Geometry check sheet. Reference: the model listing, model coordinates, mm. A direction names the side the tool comes from. Give positions to 0.01 mm unless a question says otherwise; leave off trailing zeros. Order: outer loops, then holes, each group sorted by start corner. A loop starts at its lowest first (then second) coordinate and runs counter-clockwise, first axis right, second up.
from build123d import *

# Parameters (mm, degrees)
SKETCH1_R           = 1.55
BOSS_EXTRUDE1_DEPTH = 1.5748
SKETCH2_W           = 12.4
SKETCH2_H           = 28.6
BOSS_EXTRUDE2_DEPTH = 24.9
SKETCH3_W           = 4.75
SKETCH3_H           = 0.5
BOSS_EXTRUDE3_DEPTH = 8.5
SKETCH4_W           = 45
SKETCH4_H           = 57.9
BOSS_EXTRUDE4_DEPTH = 19.1


with BuildPart() as part:
    # Sketch1 → Boss-Extrude1 (new body)
    with BuildSketch(Plane.XY):
        with BuildLine():
            Line((42.354093023, -30.703264053), (42.354093023, -32.943264053))
            Line((42.354093023, -32.943264053), (-42.354093023, -32.943264053))
            Line((-42.354093023, -32.943264053), (-42.354093023, -30.703264053))
            ThreePointArc((-42.354093023, -30.703264053), (-45.283025211, -23.632196241), (-52.354093023, -20.703264053))
            Line((-52.354093023, -20.703264053), (-60.301272865, -20.703264053))
            Line((-60.301272865, -20.703264053), (-60.301272865, 20.296735947))
            Line((-60.301272865, 20.296735947), (-52.354093023, 20.296735947))
            ThreePointArc((-52.354093023, 20.296735947), (-45.283025211, 23.225668135), (-42.354093023, 30.296735947))
            Line((-42.354093023, 30.296735947), (-42.354093023, 32.536735947))
            Line((-42.354093023, 32.536735947), (42.354093023, 32.536735947))
            Line((42.354093023, 32.536735947), (42.354093023, 30.296735947))
            ThreePointArc((42.354093023, 30.296735947), (45.283025211, 23.225668135), (52.354093023, 20.296735947))
            Line((52.354093023, 20.296735947), (54.593335979, 20.296735947))
            Line((54.593335979, 20.296735947), (54.593335979, -20.703264053))
            Line((54.593335979, -20.703264053), (52.354093023, -20.703264053))
            ThreePointArc((52.354093023, -20.703264053), (45.283025211, -23.632196241), (42.354093023, -30.703264053))
        make_face()
        with Locations((49.618335979, -15.728264053)):
            Circle(SKETCH1_R, mode=Mode.SUBTRACT)
        with Locations((49.618335979, 15.321735947)):
            Circle(SKETCH1_R, mode=Mode.SUBTRACT)
    extrude(amount=BOSS_EXTRUDE1_DEPTH)

    # Sketch2 → Boss-Extrude2 (add)
    with BuildSketch(Plane.XY.offset(1.5748)):
        with Locations((-30.457181744, 14.174173465)):
            Rectangle(SKETCH2_W, SKETCH2_H)
        with Locations((-16.057181744, 14.174173465)):
            Rectangle(SKETCH2_W, SKETCH2_H)
    extrude(amount=BOSS_EXTRUDE2_DEPTH)

    # Sketch3 → Boss-Extrude3 (add)
    with BuildSketch(Plane.XY.offset(26.4748)):
        with Locations((-16.064182879, 4.152019918)):
            Rectangle(SKETCH3_W, SKETCH3_H)
        with Locations((-16.064182879, 10.652019918)):
            Rectangle(SKETCH3_W, SKETCH3_H)
        with Locations((-30.792693371, 4.152019918)):
            Rectangle(SKETCH3_W, SKETCH3_H)
        with Locations((-30.792693371, 10.652019918)):
            Rectangle(SKETCH3_W, SKETCH3_H)
    extrude(amount=BOSS_EXTRUDE3_DEPTH)

    # Sketch4 → Boss-Extrude4 (add)
    with BuildSketch(Plane.XY.offset(1.5748)):
        with Locations((15.786645431, 0.061567403)):
            Rectangle(SKETCH4_W, SKETCH4_H)
    extrude(amount=BOSS_EXTRUDE4_DEPTH)


solid = part.part
Item 1: Sectioned sample at C-C (y = -3). Enter the section's corners in (x, z), and give its area (3 significant figures).
Reported:
outline: (-60.3, 0) - (54.59, 0) - (54.59, 1.57) - (38.29, 1.57) - (38.29, 20.67) - (-6.71, 20.67) - (-6.71, 1.57) - (-60.3, 1.57) - close
area: 1,040 mm2
Item 2: Sectioned sample at D-D (x = 30). Enter the section's corners in (y, z), and give its area (3 significant figures).
Reported:
outline: (-32.94, 0) - (32.54, 0) - (32.54, 1.57) - (29.01, 1.57) - (29.01, 20.67) - (-28.89, 20.67) - (-28.89, 1.57) - (-32.94, 1.57) - close
area: 1,210 mm2
Item 3: Draft check along X on faces 1 (the flat face through (15, 0, 20.675)), 2 (the cylindrical face through (45.361, -23.555, 0.776)), 3 (the cylindrical face through (48.07, 15.39, 0.78)). Enter one of: released by +X, released by -X, zero draft, split by the parting line, or undercut.
Reported:
face 1: zero draft
face 2: released by +X
face 3: undercut
Item 4: Gauge pin test, flat ends, axial feed: pin 1 (2 mm diameter, centred on y = -18.5, z = 5.5, fed in from -X); pin 2 (3 mm diameter, centred on y = -14, z = 10.5, fed in from +X); pin 3 (0.6 mm diameter, centred on y = 10.5, z = 31, fed in from +X); pin 4 (3 mm diameter, centred on x = 49.62, y = 15.32, fed in from +Z). Record the tip position at first contact, or that the pin passes through.
Reported:
pin 1: stops at x = -6.71
pin 2: stops at x = 38.29
pin 3: stops at x = -13.69
pin 4: passes through
Item 5: Scan lines: L1, parallel to X at y = 22, z = 3; L2, parallel to X at y = 16.5, z = 23.5; L3, parallel to Z at x = -20, y = -15.5. Record each from-to range of solid material in increasing order.
Reported:
L1: x = -36.66 to -24.26, -22.26 to -9.86, -6.71 to 38.29
L2: x = -36.66 to -24.26, -22.26 to -9.86
L3: z = 0 to 1.57
Item 6: Sectioned sample at B-B (z = 10). Enter the section's corners in (x, y).
Reported:
outline: (-36.66, -0.13) - (-24.26, -0.13) - (-24.26, 28.47) - (-36.66, 28.47) - close; (-22.26, -0.13) - (-9.86, -0.13) - (-9.86, 28.47) - (-22.26, 28.47) - close; (-6.71, -28.89) - (38.29, -28.89) - (38.29, 29.01) - (-6.71, 29.01) - close
Item 7: Set-up check for faces 4 (the flat face through (-31, -0.126, 14)), 5 (the flat face through (15, -28.888, 11)), 6 (the flat face through (-31, 4.402, 31)), 7 (the flat face through (15, 29.012, 11)): record each of +Z, -Z, +X, -X, +Y, -Y from which the full face is reachable in a straight line by a thin tool's end or side.
Reported:
face 4: +Z, -X, -Y
face 5: +Z, +X, -X, -Y
face 6: +Z, +X, -X
face 7: +Z, +X, -X, +Y
Item 8: Sectioned sample at A-A (z = 32.5). Enter the section's corners in (x, y), and give its area (3 significant figures).
Reported:
outline: (-33.17, 3.9) - (-28.42, 3.9) - (-28.42, 4.4) - (-33.17, 4.4) - close; (-33.17, 10.4) - (-28.42, 10.4) - (-28.42, 10.9) - (-33.17, 10.9) - close; (-18.44, 3.9) - (-13.69, 3.9) - (-13.69, 4.4) - (-18.44, 4.4) - close; (-18.44, 10.4) - (-13.69, 10.4) - (-13.69, 10.9) - (-18.44, 10.9) - close
area: 9.50 mm2
